```python
from build123d import *

# Parameters (mm, degrees)
BOSS_EXTRUDE3_DEPTH     = 20.32
BOSS_EXTRUDE4_DEPTH     = 2.54
FILLET2_R               = 2.54
SKETCH3_R               = 1.905
CUT_EXTRUDE2_DEPTH      = 51.8
CUT_EXTRUDE2_DEPTH_BACK = 1


with BuildPart() as part:
    # Sketch2 → Boss-Extrude3 (new body)
    with BuildSketch(Plane.XY):
        with BuildLine():
            Line((24.13, 37.9095), (24.13, 0))
            Line((24.13, 0), (28.557757617, 0))
            Line((28.557757617, 0), (28.557757617, 36.423556552))
            ThreePointArc((28.557757617, 36.423556552), (42.3545, 54.102), (28.557757617, 71.780443448))
            Line((28.557757617, 71.780443448), (28.557757617, 82.55))
            Line((28.557757617, 82.55), (24.13, 82.55))
            Line((24.13, 82.55), (24.13, 70.2945))
            ThreePointArc((24.13, 70.2945), (35.579826554, 65.551826554), (40.3225, 54.102))
            ThreePointArc((40.3225, 54.102), (35.579826554, 42.652173446), (24.13, 37.9095))
        make_face()
    extrude(amount=BOSS_EXTRUDE3_DEPTH)

    # Sketch2<5> → Boss-Extrude4 (add)
    with BuildSketch(Plane.XY):
        with BuildLine():
            Line((28.557757617, 36.423556552), (28.557757617, 0))
            Line((28.557757617, 0), (50.8, 0))
            Line((50.8, 0), (50.8, 82.55))
            Line((50.8, 82.55), (28.557757617, 82.55))
            Line((28.557757617, 82.55), (28.557757617, 71.780443448))
            ThreePointArc((28.557757617, 71.780443448), (42.3545, 54.102), (28.557757617, 36.423556552))
        make_face()
    extrude(amount=BOSS_EXTRUDE4_DEPTH)

    # Fillet2
    fillet2_edges = [part.edges().sort_by_distance(p)[0] for p in [
        (42.3545, 54.102, 2.54),
        (28.557757617, 18.211778276, 2.54),
        (28.557757617, 77.165221724, 2.54),
    ]]
    fillet(fillet2_edges, radius=FILLET2_R)

    # Sketch3 → Cut-Extrude2 (cut, two sides)
    with BuildSketch(Plane(origin=(0, 0, 0), x_dir=(0, 0, -1), z_dir=(1, 0, 0))) as cut_extrude2_sk:
        with Locations((-12.7, 18.430889618)):
            Circle(SKETCH3_R)
        with Locations((-12.7, 76.946110382)):
            Circle(SKETCH3_R)
    extrude(amount=CUT_EXTRUDE2_DEPTH, mode=Mode.SUBTRACT)
    extrude(cut_extrude2_sk.sketch, amount=-CUT_EXTRUDE2_DEPTH_BACK, mode=Mode.SUBTRACT)


solid = part.part
```
Source: CAD feature listing. Evaluate the final solid. Frame: model axes, mm. A direction names the side the tool comes from. Round coordinates to 2 decimals unless told otherwise and drop trailing zeros. Write each loop counter-clockwise with the first axis right and the second up, starting at its lowest first coordinate (ties: lowest second). Pieces come first, ordered by that corner, then holes. Notation, with made-up numbers: M -10.75,1 L 21.25,1 A22 ccw 21.25,32 Z; hole C 6.25,0.5 d2. An arc over 180 degrees is marked long. Use CSV: the item, a comma, the result in double quotes. Start each with the question number.
Q1. Cut plane B-B on y = 6.5. Output: boundary loops of the cut face in (x, z), plus the area to 3 significant figures.
Q2. Pull-direction query (Z, two-part tool) for faces 6 (the face through (24.13, 19, 10)), 7 (the face through (30, 38, 20.32)), 8 (the face through (26.313, 75.086, 13.113)); classes: +Z half, -Z half, draft (parallel to the pull), parting line (faces both ways), or undercut.
Q3. First-contact query: P1, Ø5, axis at y = 55, z = 17.5, coming from the -X side; P2, Ø6, axis at y = 55, z = 6.5, coming from the +X side; P3, Ø6, axis at x = 38.5, y = 25, coming from the +Z side. Flat tips, straight axial feed; report the tip coordinate or a pass-through.
Q4. Cut plane A-A on z = 12.7. Count the separate pieces of the cut face and the enclosed holes in it, plus the area to 3 significant figures.
Q5. Access query for faces 1 (the face through (26.31, 20.32, 12.95)), 2 (the face through (43, 42, 2.54)), 3 (the face through (50.8, 41, 1)), 4 (the face through (28.558, 78.3, 10.9)), 5 (the face through (28.558, 18, 9)). Directions: +Z, -Z, +X, -X, +Y, -Y. A direction counts if a zero-diameter tool reaches every point of the face in a straight line with its end or side. Return the directions, or none.
Q6. Cut plane C-C on x = 47.25. Output: boundary loops of the cut face in (y, z).
Q7. Line query: line 1 (Y direction, x = 27.3, z = 12.7); line 2 (Y direction, x = 26.65, z = 12.7); line 3 (X direction, y = 78, z = 9.25). Output: solid intervals per line, ascending. Write a range as from..to.
Results found:
1,outline,"M 24.13,0 L 50.8,0 L 50.8,2.54 L 31.1,2.54 A2.54 cw 28.56,5.08 L 28.56,20.32 L 24.13,20.32 Z"
1,area,"148 mm^2"
2,face 6,"draft"
2,face 7,"+Z half"
2,face 8,"undercut"
3,P1,"x = 39.96"
3,P2,"x = 42.89"
3,P3,"z = 2.54"
4,separate pieces,"3"
4,enclosed holes,"0"
4,area,"282 mm^2"
5,face 1,"+X, -X"
5,face 2,"+Z, +X"
5,face 3,"+Z, -Z, +X, +Y, -Y"
5,face 4,"+Z, +X, +Y"
5,face 5,"+Z, +X, -Y"
6,outline,"M 0,0 L 82.55,0 L 82.55,2.54 L 0,2.54 Z"
7,line 1,"0..16.53, 20.34..38.22, 69.98..75.04, 78.85..82.55"
7,line 2,"0..16.53, 20.34..38.11, 70.1..75.04, 78.85..82.55"
7,line 3,"24.13..28.56"
